Could you check a few things on this model? Use its own coordinates, in mm. A direction names the side the tool comes from. Give positions to 0.01 mm unless a question says otherwise; leave off trailing zeros. Order: outer loops, then holes, each group sorted by start corner. A loop starts at its lowest first (then second) coordinate and runs counter-clockwise, first axis right, second up.
(1) Imagine slicing it at D-D, the plane x = -11.4. Write out the boundary of the cut face in (y, z).
(2) Imagine slicing it at C-C, the plane z = 7.25. Write out the boundary of the cut face in (x, y), then the cut area to 3 significant figures.
(3) Will these pins go through, and if not, where does the flat tip stop? pin 1 (2 mm diameter, centred on y = -19, z = 10.5, fed in from +X); pin 2 (4 mm diameter, centred on x = 10.5, z = 5.5, fed in from +Y); pin 3 (2 mm diameter, centred on y = 16.5, z = 11.5, fed in from -X).
(4) If I drill on probe 1 along Y at (x, z) = (-18, 1.5); probe 2 along X at (y, z) = (-8.5, 3.5); probe 3 along Y at (x, z) = (9.5, 10.5), over which ranges is the centre line in solid material (lowest first)?
(5) Imagine slicing it at B-B, the plane x = 10.7. Write out the boundary of the cut face in (y, z).
(6) Imagine slicing it at A-A, the plane y = 0. Write out the boundary of the cut face in (x, z).
(7) If we mould it in two halves opening along X, with no side actions, what happens to faces 1 (the flat face through (0, -14, 13)), 2 (the flat face through (15, 17, 11)), 3 (the flat face through (0, 0, 1))? For each: released by +X, released by -X, zero draft, split by the parting line, or undercut.
(8) On a 3-axis mill with a long thin cutter (end or side, diameter ignored), from which of +Z, -Z, +X, -X, +Y, -Y can I reach the whole of each face in a straight line? I mean faces 4 (the flat face through (0, -13.5, 10)), 5 (the flat face through (0, 0, 0)), 6 (the flat face through (0, 17, 11)), 7 (the flat face through (0, -18, 11)), 8 (the flat face through (9, 18, 9)). Say none if no direction works.
from build123d import *

# Parameters (mm, degrees)
SKETCH1_W           = 53
SKETCH1_H           = 29
BOSS_EXTRUDE2_DEPTH = 13
SHELL5_T            = -1
SKETCH3_R           = 8.25
CUT_EXTRUDE1_DEPTH  = 13
SKETCH4_W           = 10
SKETCH4_H           = 5.3
CUT_EXTRUDE2_DEPTH  = 13
SKETCH5_W           = 15
SKETCH5_H           = 6
BOSS_EXTRUDE3_DEPTH = 4
SKETCH6_R           = 1.75
CUT_EXTRUDE3_DEPTH  = 6


with BuildPart() as part:
    # Sketch1 → Boss-Extrude2 (new body)
    with BuildSketch(Plane.XY):
        Rectangle(SKETCH1_W, SKETCH1_H)
    extrude(amount=BOSS_EXTRUDE2_DEPTH)

    # Shell5
    shell5_openings = [part.faces().sort_by_distance(p)[0] for p in [
        (0, 0, 13),
    ]]
    offset(amount=SHELL5_T, openings=shell5_openings, kind=Kind.INTERSECTION)

    # Sketch3 → Cut-Extrude1 (cut)
    with BuildSketch(Plane.XY.offset(1)):
        with Locations((-11.4, 0)):
            Circle(SKETCH3_R)
        with Locations((10.7, 0)):
            Circle(SKETCH3_R)
    extrude(amount=-CUT_EXTRUDE1_DEPTH, mode=Mode.SUBTRACT)

    # Sketch4 → Cut-Extrude2 (cut)
    with BuildSketch(Plane.XZ.offset(14.5)):
        with Locations((1, 6.35)):
            Rectangle(SKETCH4_W, SKETCH4_H)
    extrude(amount=-CUT_EXTRUDE2_DEPTH, mode=Mode.SUBTRACT)

    # Sketch5 → Boss-Extrude3 (add)
    with BuildSketch(Plane.XY.offset(13)):
        with Locations((7.5, 17.5)):
            Rectangle(SKETCH5_W, SKETCH5_H)
        with Locations((7.5, -17.5)):
            Rectangle(SKETCH5_W, SKETCH5_H)
    extrude(amount=-BOSS_EXTRUDE3_DEPTH)

    # Sketch6 → Cut-Extrude3 (cut)
    with BuildSketch(Plane.XY.offset(13)):
        with Locations((6.914840987, 17.533686801)):
            Circle(SKETCH6_R)
        with Locations((6.914840987, -17.647083132)):
            Circle(SKETCH6_R)
    extrude(amount=-CUT_EXTRUDE3_DEPTH, mode=Mode.SUBTRACT)


solid = part.part
Answer block:
1. outline: (-14.5, 0) - (-8.25, 0) - (-8.25, 1) - (-13.5, 1) - (-13.5, 13) - (-14.5, 13) - close; (8.25, 0) - (14.5, 0) - (14.5, 13) - (13.5, 13) - (13.5, 1) - (8.25, 1) - close
2. outline: (-26.5, -14.5) - (-4, -14.5) - (-4, -13.5) - (-25.5, -13.5) - (-25.5, 13.5) - (25.5, 13.5) - (25.5, -13.5) - (6, -13.5) - (6, -14.5) - (26.5, -14.5) - (26.5, 14.5) - (-26.5, 14.5) - close
2. area: 150 mm2
3. pin 1: stops at x = 15
3. pin 2: stops at y = 14.5
3. pin 3: stops at x = 0
4. probe 1: y = -14.5 to -13.5, 13.5 to 14.5
4. probe 2: x = -26.5 to -25.5, 25.5 to 26.5
4. probe 3: y = -20.5 to -13.5, 13.5 to 20.5
5. outline: (-20.5, 9) - (-14.5, 9) - (-14.5, 0) - (-8.25, 0) - (-8.25, 1) - (-13.5, 1) - (-13.5, 13) - (-20.5, 13) - close; (8.25, 0) - (14.5, 0) - (14.5, 9) - (20.5, 9) - (20.5, 13) - (13.5, 13) - (13.5, 1) - (8.25, 1) - close
6. outline: (-26.5, 0) - (-19.65, 0) - (-19.65, 1) - (-25.5, 1) - (-25.5, 13) - (-26.5, 13) - close; (-3.15, 0) - (2.45, 0) - (2.45, 1) - (-3.15, 1) - close; (18.95, 0) - (26.5, 0) - (26.5, 13) - (25.5, 13) - (25.5, 1) - (18.95, 1) - close
7. face 1: zero draft
7. face 2: released by +X
7. face 3: undercut
8. face 4: +Z
8. face 5: -Z, +X, -X, +Y, -Y
8. face 6: +Z, -Z, -X, +Y
8. face 7: +Z, -Z, -X, -Y
8. face 8: -Z, +X, -X, +Y
